Part model, mm, in its own coordinate system. A direction names the side the tool comes from. Round coordinates to 2 decimals unless told otherwise and drop trailing zeros. Order: outer loops, then holes, each group sorted by start corner. A loop starts at its lowest first (then second) coordinate and runs counter-clockwise, first axis right, second up. Notation, with made-up numbers: (46.25, -39) -> (76.25, -39) arc R15 ccw to (76.25, -25) -> close; hole circle Ø9 at (13.25, 65). An arc over 180 degrees is marked (long way). Answer as a JSON object with one key per item and string values. Group by question number.
```python
from build123d import *

# Parameters (mm, degrees)
F0_W          = 150
F0_H          = 12
F1_DEPTH      = 3
F1_DEPTH_BACK = 2
F2_R          = 2.25
F3_DEPTH      = 29
F4_START      = -36
F4_DEPTH      = 78
F5_START      = -121
F5_DEPTH      = 29


with BuildPart() as f1:
    # F0 (on Top) → F1 (new body, two sides)
    with BuildSketch(Plane.XY) as f1_sk:
        with Locations((75, 6)):
            Rectangle(F0_W, F0_H)
    extrude(amount=F1_DEPTH)
    extrude(f1_sk.sketch, amount=-F1_DEPTH_BACK)

    # F2 (on face) → F3 (join)
    with BuildSketch(Plane(origin=(0, 0, 0), x_dir=(0, -1, 0), z_dir=(-1, 0, 0))):
        with BuildLine():
            Line((-12, 5), (-12, 3))
            Line((-12, 3), (0, 3))
            Line((0, 3), (0, 5))
            ThreePointArc((0, 5), (-6, 11), (-12, 5))
        make_face()
        with Locations((-6, 7)):
            Circle(F2_R, mode=Mode.SUBTRACT)
    extrude(amount=-F3_DEPTH)

    # F2 (on face) → F4 (join)
    with BuildSketch(Plane(origin=(0, 0, 0), x_dir=(0, -1, 0), z_dir=(-1, 0, 0)).offset(F4_START)):
        with BuildLine():
            Line((-12, 5), (-12, 3))
            Line((-12, 3), (0, 3))
            Line((0, 3), (0, 5))
            ThreePointArc((0, 5), (-6, 11), (-12, 5))
        make_face()
        with Locations((-6, 7)):
            Circle(F2_R, mode=Mode.SUBTRACT)
    extrude(amount=-F4_DEPTH)

    # F2 (on face) → F5 (join)
    with BuildSketch(Plane(origin=(0, 0, 0), x_dir=(0, -1, 0), z_dir=(-1, 0, 0)).offset(F5_START)):
        with BuildLine():
            Line((-12, 5), (-12, 3))
            Line((-12, 3), (0, 3))
            Line((0, 3), (0, 5))
            ThreePointArc((0, 5), (-6, 11), (-12, 5))
        make_face()
        with Locations((-6, 7)):
            Circle(F2_R, mode=Mode.SUBTRACT)
    extrude(amount=-F5_DEPTH)


solid = f1.part
```
Q1. Wall check: line 1 (X direction, y = 2, z = 8); line 2 (Z direction, x = 131, y = 6); line 3 (Y direction, x = 134.5, z = 7.5). Give the ranges that are in metal, low to high. Write a range as [from, to].
Q2. Two-plate mould, pull along Z, no slides. Class faces 3 (the cylindrical face through (74, 6, 11)), 4 (the cylindrical face through (135.297, 4.79, 8.897)), 5 (the flat face through (36, 6, 4)): +Z half, -Z half, draft (parallel to the pull), parting line (faces both ways), or undercut.
Q3. Band-saw the part on B-B (x = 82.5). List the corners of the cut face in (y, z), plus the area to 3 significant figures.
Q4. Band-saw the part on C-C (z = 7). List the corners of the cut face in (x, y), plus the area to 3 significant figures.
Q5. Band-saw the part on A-A (y = 6). List the corners of the cut face in (x, z).
Q6. Which spindle directions (+Z, -Z, +X, -X, +Y, -Y) get a long thin tool onto all of the face, cutting with end or side? Do faces 1 (the flat face through (32, 6, 3)), 2 (the cylindrical face through (135, 6, 11)). Say none if no direction does.
Q7. Drop flat-ended pins along their axis: pin 1 Ø4 at (x, z) = (135, 9) entering from +Y; pin 2 Ø5.5 at (x, y) = (118, 4) entering from +Z. Give the stop position or say it passes through.
Completed:
{
 "1": {"line 1": "[0, 29], [36, 114], [121, 150]", "line 2": "[-2, 4.75], [9.25, 11]", "line 3": "[0.55, 3.81], [8.19, 11.45]"},
 "2": {"face 3": "+Z half", "face 4": "undercut", "face 5": "draft"},
 "3": {"outline": "(0, -2) -> (12, -2) -> (12, 5) arc R6 ccw to (0, 5) -> close; hole circle Ø4.5 at (6, 7)", "area": "125 mm2"},
 "4": {"outline": "(0, 0.34) -> (29, 0.34) -> (29, 3.75) -> (0, 3.75) -> close; (0, 8.25) -> (29, 8.25) -> (29, 11.66) -> (0, 11.66) -> close; (36, 0.34) -> (114, 0.34) -> (114, 3.75) -> (36, 3.75) -> close; (36, 8.25) -> (114, 8.25) -> (114, 11.66) -> (36, 11.66) -> close; (121, 0.34) -> (150, 0.34) -> (150, 3.75) -> (121, 3.75) -> close; (121, 8.25) -> (150, 8.25) -> (150, 11.66) -> (121, 11.66) -> close", "area": "927 mm2"},
 "5": {"outline": "(0, -2) -> (150, -2) -> (150, 4.75) -> (121, 4.75) -> (121, 3) -> (114, 3) -> (114, 4.75) -> (36, 4.75) -> (36, 3) -> (29, 3) -> (29, 4.75) -> (0, 4.75) -> close; (0, 9.25) -> (29, 9.25) -> (29, 11) -> (0, 11) -> close; (36, 9.25) -> (114, 9.25) -> (114, 11) -> (36, 11) -> close; (121, 9.25) -> (150, 9.25) -> (150, 11) -> (121, 11) -> close"},
 "6": {"face 1": "+Z, +Y, -Y", "face 2": "+Z, +X, -X"},
 "7": {"pin 1": "y = 11.66", "pin 2": "z = 3"}
}
